Part model, mm, in its own coordinate system. A direction names the side the tool comes from. Round coordinates to 2 decimals unless told otherwise and drop trailing zeros. Loops run counter-clockwise (first coordinate to the right, second up) from the corner with the lowest first, then second, coordinate; pieces in that order, holes last. Notation, with made-up numbers: M 63,28 L 101,28 A15 cw 101,51 Z; hole C 16.25,15.5 d8. An arc over 180 degrees is marked long. Answer as CSV lines item,"result". Start each with the question number.
Item 1: Band-saw the part on B-B (z = 0). Give the cut face in (x, y), and give its area (3 significant figures).
Item 2: Band-saw the part on D-D (y = 18.5). Give the cut face in (x, z).
Item 3: Wall check: line 1 (X direction, y = 8.25, z = 0); line 2 (Y direction, x = -1.5, z = -7.25); line 3 (X direction, y = 6.25, z = 1.25). Give the ranges that are in metal, low to high.
Item 4: Band-saw the part on A-A (x = 0). Give the cut face in (y, z).
Item 5: Drop flat-ended pins along their axis: pin 1 Ø1 at (x, z) = (0.5, -6.5) entering from +Y; pin 2 Ø8 at (x, y) = (6, 5.5) entering from -Z; pin 3 Ø1.5 at (y, z) = (11, -3) entering from -X. Give the stop position or say it passes through.
Item 6: Mould opens along Z. For faces 3 (the cylindrical face through (-7.81, 16.2, -1.73)), 4 (the cylindrical face through (-3.543, 14.79, 8.545)), 5 (the flat face through (2.2, 0, -0.1)) say: pulls with the +Z half, pulls with the -Z half, needs draft (parallel to the pull), parting line crosses it, or undercut.
Item 7: Band-saw the part on C-C (z = 3.25). Give the cut face in (x, y).
Item 8: Which spindle directions (+Z, -Z, +X, -X, +Y, -Y) get a long thin tool onto all of the face, cutting with end or side? Do faces 1 (the flat face through (-2, 2, 2)), 2 (the flat face through (8, 30, -3)). Say none if no direction does.
```python
from build123d import *

# Parameters (mm, degrees)
SKETCH1_R               = 9.25
BOSS_EXTRUDE1_DEPTH     = 30
CUT_EXTRUDE1_START      = 30
SKETCH1_3_R             = 8
CUT_EXTRUDE1_DEPTH      = 28
CUT_EXTRUDE3_DEPTH      = 33.728046077
CUT_EXTRUDE3_DEPTH_BACK = 33.728046077
SKETCH1_4_R             = 2


with BuildPart() as part:
    # Sketch1 → Boss-Extrude1 (new body)
    with BuildSketch(Plane(origin=(0, 0, 0), x_dir=(1, 0, 0), z_dir=(0, 1, 0))):
        with Locations(Location((0, 0, 0), (0, 0, 270))):
            Circle(SKETCH1_R)
    extrude(amount=BOSS_EXTRUDE1_DEPTH)

    # Sketch1<3> → Cut-Extrude1 (cut)
    with BuildSketch(Plane(origin=(0, 0, 0), x_dir=(1, 0, 0), z_dir=(0, 1, 0)).offset(CUT_EXTRUDE1_START)):
        with Locations(Location((0, 0, 0), (0, 0, 270))):
            Circle(SKETCH1_3_R)
    extrude(amount=-CUT_EXTRUDE1_DEPTH, mode=Mode.SUBTRACT)

    # Sketch1<4> → Cut-Extrude3 (cut, two sides: drawn at the far end of the back side and taken through both)
    with BuildSketch(Plane(origin=(0, 0, 0), x_dir=(1, 0, 0), z_dir=(0, 1, 0)).offset(-CUT_EXTRUDE3_DEPTH_BACK)):
        with Locations(Location((0, 0, 0), (0, 0, 270))):
            Circle(SKETCH1_4_R)
    extrude(amount=CUT_EXTRUDE3_DEPTH + CUT_EXTRUDE3_DEPTH_BACK, mode=Mode.SUBTRACT)


solid = part.part
```
Answer block:
1,outline,"M -9.25,0 L -2,0 L -2,2 L -8,2 L -8,30 L -9.25,30 Z; M 2,0 L 9.25,0 L 9.25,30 L 8,30 L 8,2 L 2,2 Z"
1,area,"99.0 mm^2"
2,outline,"C 0,0 d18.5; hole C 0,0 d16"
3,line 1,"x = -9.25 to -8, 8 to 9.25"
3,line 2,"y = 0 to 2"
3,line 3,"x = -9.17 to -7.9, 7.9 to 9.17"
4,outline,"M 0,-9.25 L 30,-9.25 L 30,-8 L 2,-8 L 2,-2 L 0,-2 Z; M 0,2 L 2,2 L 2,8 L 30,8 L 30,9.25 L 0,9.25 Z"
5,pin 1,"stops at y = 2"
5,pin 2,"stops at z = -9.03"
5,pin 3,"stops at x = -8.97"
6,face 3,"undercut"
6,face 4,"parting line crosses it"
6,face 5,"needs draft"
7,outline,"M -8.66,0 L 8.66,0 L 8.66,30 L 7.31,30 L 7.31,2 L -7.31,2 L -7.31,30 L -8.66,30 Z"
8,face 1,"+Y"
8,face 2,"+Z, -Z, +X, -X, +Y"
